```python
from build123d import *

# Parameters (mm, degrees)
F0_W     = 606.425
F0_H     = 279.4
F1_DEPTH = 3.175
F2_W     = 107.95
F2_H     = 82.55
F3_DEPTH = 38.1
F4_DEPTH = 1.5875
F5_W     = 101.6
F5_H     = 76.2
F6_DEPTH = 38.1


with BuildPart() as f1:
    # F0 (on Front) → F1 (new body)
    with BuildSketch(Plane.XZ):
        Rectangle(F0_W, F0_H)
    extrude(amount=F1_DEPTH)

    # F2 (on face) → F3 (join)
    with BuildSketch(Plane.XZ.offset(3.175)):
        with Locations((0, 73.025)):
            Rectangle(F2_W, F2_H)
    extrude(amount=-F3_DEPTH)

    # F2 (on face) → F4 (join)
    with BuildSketch(Plane.XZ.offset(3.175)):
        with Locations((0, 73.025)):
            Rectangle(F2_W, F2_H)
    extrude(amount=F4_DEPTH)

    # F5 (on face) → F6 (cut)
    with BuildSketch(Plane.XZ.offset(4.7625)):
        with Locations((0, 73.025)):
            Rectangle(F5_W, F5_H)
    extrude(amount=-F6_DEPTH, mode=Mode.SUBTRACT)


solid = f1.part
```
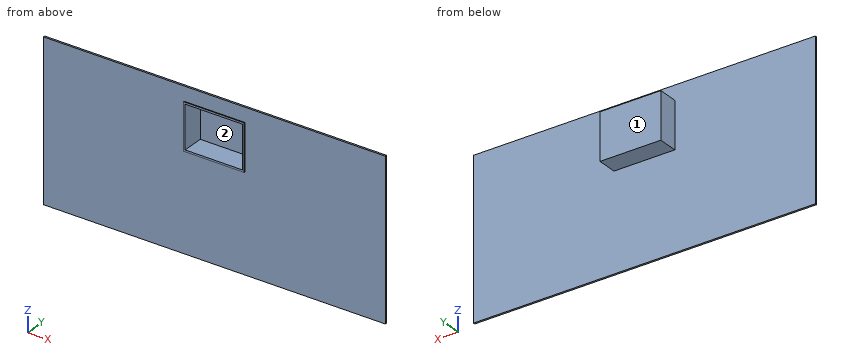
Work out the finished part from the listing and answer in its coordinate system (mm). Face numbers are marked on the shaded views. Round coordinates to 2 decimals unless told otherwise and drop trailing zeros. Loops run counter-clockwise (first coordinate to the right, second up) from the corner with the lowest first, then second, coordinate; pieces in that order, holes last. Notation, with made-up numbers: (45.25, 89) -> (81.25, 89) arc R38 ccw to (81.25, 128) -> close; hole circle Ø6 at (6.5, -29). An arc over 180 degrees is marked (long way). Write each question's results on one line, items separated by ' | '. Start each with the question number.
1. For a pull along X with two mould halves and no side action, classify the marked faces 1 and 2 as +X half, -X half, draft (parallel to the pull), parting line (faces both ways), or undercut.
2. Section D-D (z = -40) is taken. Determine the outline of the cut face in (x, y) (1 decimal).
3. Find the intervals of material crossed by probe 1 along Z at (x, y) = (-22, 22) (3 decimals); probe 2 along Y at (x, z) = (-143, -8) (3 decimals); probe 3 along X at (y, z) = (26, 107) (3 decimals), in increasing order. Write a range as from..to.
4. Section C-C (z = 83.5) is taken. Determine the outline of the cut face in (x, y) (1 decimal).
5. Section A-A (y = 20) is taken. Determine the outline of the cut face in (x, z) (3 decimals), plus the area to 3 significant figures.
6. Given pin 1 Ø10.5 at (y, z) = (16.5, 59.5) entering from +X (3 decimals); pin 2 Ø6 at (y, z) = (18.5, 53.5) entering from -X (3 decimals); pin 3 Ø11.5 at (x, y) = (-24, 9.5) entering from -Z, each flat-ended and moving along its own axis, determine where each tip first touches the part or whether it passes through.
Evaluation:
1) face 1: draft | face 2: undercut
2) outline: (-303.2, -3.2) -> (303.2, -3.2) -> (303.2, 0) -> (-303.2, 0) -> close
3) probe 1: z = 31.75..34.925, 111.125..114.3 | probe 2: y = -3.175..0 | probe 3: x = -53.975..-50.8, 50.8..53.975
4) outline: (-303.2, -3.2) -> (-54, -3.2) -> (-54, -4.8) -> (-50.8, -4.8) -> (-50.8, 33.3) -> (50.8, 33.3) -> (50.8, -4.8) -> (54, -4.8) -> (54, -3.2) -> (303.2, -3.2) -> (303.2, 0) -> (54, 0) -> (54, 34.9) -> (-54, 34.9) -> (-54, 0) -> (-303.2, 0) -> close
5) outline: (-53.975, 31.75) -> (53.975, 31.75) -> (53.975, 114.3) -> (-53.975, 114.3) -> close; hole (-50.8, 34.925) -> (50.8, 34.925) -> (50.8, 111.125) -> (-50.8, 111.125) -> close | area: 1,170 mm2
6) pin 1: stops at x = 53.975 | pin 2: stops at x = -53.975 | pin 3: stops at z = 31.75
